```python
from build123d import *

# Parameters (mm, degrees)
SKETCH_1_W          = 124
SKETCH_1_H          = 65
EXTRUDE_1_DEPTH     = 18.5
SKETCH_2_R          = 1.5
CUT_EXTRUDE_1_DEPTH = 3
SKETCH_3_W          = 14
SKETCH_3_H          = 7
SKETCH_3_W_2        = 12
SKETCH_3_H_2        = 2
CUT_EXTRUDE_2_DEPTH = 3
SKETCH_4_R          = 0.5
CUT_EXTRUDE_3_DEPTH = 3
FILLET_1_R          = 2
FILLET_2_R          = 2
FILLET_3_R          = 2
FILLET_4_R          = 2


with BuildPart() as part:
    # Эскиз1 → Бобышка-Вытянуть1 (new body)
    with BuildSketch(Plane(origin=(0, 0, 0), x_dir=(1, 0, 0), z_dir=(0, 1, 0))):
        with Locations((62, 32.5)):
            Rectangle(SKETCH_1_W, SKETCH_1_H)
    extrude(amount=EXTRUDE_1_DEPTH)

    # Эскиз2 → Вырез-Вытянуть1 (cut)
    with BuildSketch(Plane(origin=(124, 0, 0), x_dir=(0, 0, -1), z_dir=(1, 0, 0))):
        with BuildLine():
            Line((11, 14.25), (21, 14.25))
            ThreePointArc((21, 14.25), (26, 9.25), (21, 4.25))
            Line((21, 4.25), (11, 4.25))
            ThreePointArc((11, 4.25), (6, 9.25), (11, 14.25))
        make_face()
        with Locations((11, 9.25)):
            Circle(SKETCH_2_R, mode=Mode.SUBTRACT)
        with Locations((21, 9.25)):
            Circle(SKETCH_2_R, mode=Mode.SUBTRACT)
    extrude(amount=-CUT_EXTRUDE_1_DEPTH, mode=Mode.SUBTRACT)

    # Эскиз3 → Вырез-Вытянуть2 (cut)
    with BuildSketch(Plane.ZY):
        with Locations((-52, 9.25)):
            Rectangle(SKETCH_3_W, SKETCH_3_H)
        with Locations((-52, 7.75)):
            Rectangle(SKETCH_3_W_2, SKETCH_3_H_2, mode=Mode.SUBTRACT)
    extrude(amount=-CUT_EXTRUDE_2_DEPTH, mode=Mode.SUBTRACT)

    # Эскиз4 → Вырез-Вытянуть3 (cut)
    with BuildSketch(Plane.ZY):
        Polygon((-19, 9.25), (-16, 12.25), (-10, 12.25), (-7, 9.25), (-10, 6.25), (-16, 6.25), align=None)
        with Locations((-16, 9.25)):
            Circle(SKETCH_4_R, mode=Mode.SUBTRACT)
        with Locations((-14, 9.25)):
            Circle(SKETCH_4_R, mode=Mode.SUBTRACT)
        with Locations((-12, 9.25)):
            Circle(SKETCH_4_R, mode=Mode.SUBTRACT)
        with Locations((-10, 9.25)):
            Circle(SKETCH_4_R, mode=Mode.SUBTRACT)
    extrude(amount=-CUT_EXTRUDE_3_DEPTH, mode=Mode.SUBTRACT)

    # Скругление1
    fillet_1_edges = [part.edges().sort_by_distance(p)[0] for p in [
        (124, 18.5, -32.5),
        (62, 18.5, -65),
        (0, 18.5, -32.5),
        (62, 18.5, 0),
    ]]
    fillet(fillet_1_edges, radius=FILLET_1_R)

    # Скругление2
    fillet_2_edges = [part.edges().sort_by_distance(p)[0] for p in [
        (62, 0, -65),
        (124, 0, -32.5),
        (62, 0, 0),
        (0, 0, -32.5),
    ]]
    fillet(fillet_2_edges, radius=FILLET_2_R)

    # Скругление3
    # the kernel refuses this fillet: 2 mm, written as the material it takes off along each edge
    with BuildSketch(Plane(origin=(2, 16.5, -2), x_dir=(-1, 0, 0), z_dir=(0, 0, 1))) as fillet_3_piece_1_section:
        Polygon((0, 0), (FILLET_3_R, 0), (FILLET_3_R, -FILLET_3_R), (0, -FILLET_3_R), align=None)
    fillet_3_piece_1 = extrude(amount=FILLET_3_R, mode=Mode.PRIVATE)
    fillet_3_piece_1 = fillet_3_piece_1 - Plane(origin=(2, 16.5, -2), x_dir=(0.7071067811865475, -0.7071067811865475, 0), z_dir=(0, 0, 1)) * Sphere(FILLET_3_R, mode=Mode.PRIVATE)
    add(fillet_3_piece_1, mode=Mode.SUBTRACT)
    with BuildSketch(Plane(origin=(122, 16.5, -2), x_dir=(1, 0, 0), z_dir=(0, 0, 1))) as fillet_3_piece_2_section:
        Polygon((0, 0), (FILLET_3_R, 0), (FILLET_3_R, FILLET_3_R), (0, FILLET_3_R), align=None)
    fillet_3_piece_2 = extrude(amount=FILLET_3_R, mode=Mode.PRIVATE)
    fillet_3_piece_2 = fillet_3_piece_2 - Plane(origin=(122, 16.5, -2), x_dir=(-0.7071067811865475, -0.7071067811865475, 0), z_dir=(0, 0, 1)) * Sphere(FILLET_3_R, mode=Mode.PRIVATE)
    add(fillet_3_piece_2, mode=Mode.SUBTRACT)
    with BuildSketch(Plane(origin=(2, 2, -2), x_dir=(-1, 0, 0), z_dir=(0, 0, 1))) as fillet_3_piece_3_section:
        Polygon((0, 0), (FILLET_3_R, 0), (FILLET_3_R, FILLET_3_R), (0, FILLET_3_R), align=None)
    fillet_3_piece_3 = extrude(amount=FILLET_3_R, mode=Mode.PRIVATE)
    fillet_3_piece_3 = fillet_3_piece_3 - Plane(origin=(2, 2, -2), x_dir=(0.7071067811865475, 0.7071067811865475, 0), z_dir=(0, 0, 1)) * Sphere(FILLET_3_R, mode=Mode.PRIVATE)
    add(fillet_3_piece_3, mode=Mode.SUBTRACT)
    with BuildSketch(Plane(origin=(122, 2, -2), x_dir=(1, 0, 0), z_dir=(0, 0, 1))) as fillet_3_piece_4_section:
        Polygon((0, 0), (FILLET_3_R, 0), (FILLET_3_R, -FILLET_3_R), (0, -FILLET_3_R), align=None)
    fillet_3_piece_4 = extrude(amount=FILLET_3_R, mode=Mode.PRIVATE)
    fillet_3_piece_4 = fillet_3_piece_4 - Plane(origin=(122, 2, -2), x_dir=(-0.7071067811865475, 0.7071067811865475, 0), z_dir=(0, 0, 1)) * Sphere(FILLET_3_R, mode=Mode.PRIVATE)
    add(fillet_3_piece_4, mode=Mode.SUBTRACT)
    with BuildSketch(Plane(origin=(124, 2, 0), x_dir=(-1, 0, 0), z_dir=(0, 1, 0))) as fillet_3_piece_5:
        with BuildLine():
            CenterArc((FILLET_3_R, -FILLET_3_R), FILLET_3_R, 90, 90)
            Line((0, -FILLET_3_R), (0, 0))
            Line((0, 0), (FILLET_3_R, 0))
        make_face()
    extrude(amount=14.5, mode=Mode.SUBTRACT)
    with BuildSketch(Plane(origin=(0, 2, 0), x_dir=(1, 0, 0), z_dir=(0, 1, 0))) as fillet_3_piece_6:
        with BuildLine():
            CenterArc((FILLET_3_R, FILLET_3_R), FILLET_3_R, 180, 90)
            Line((0, FILLET_3_R), (0, 0))
            Line((0, 0), (FILLET_3_R, 0))
        make_face()
    extrude(amount=14.5, mode=Mode.SUBTRACT)

    # Скругление4
    # the kernel refuses this fillet: 2 mm, written as the material it takes off along each edge
    with BuildSketch(Plane(origin=(2, 16.5, -63), x_dir=(0, 0, -1), z_dir=(-1, 0, 0))) as fillet_4_piece_1_section:
        Polygon((0, 0), (FILLET_4_R, 0), (FILLET_4_R, -FILLET_4_R), (0, -FILLET_4_R), align=None)
    fillet_4_piece_1 = extrude(amount=FILLET_4_R, mode=Mode.PRIVATE)
    fillet_4_piece_1 = fillet_4_piece_1 - Plane(origin=(2, 16.5, -63), x_dir=(0, -0.7071067811865475, 0.7071067811865475), z_dir=(-1, 0, 0)) * Sphere(FILLET_4_R, mode=Mode.PRIVATE)
    add(fillet_4_piece_1, mode=Mode.SUBTRACT)
    with BuildSketch(Plane(origin=(122, 16.5, -63), x_dir=(0, 0, -1), z_dir=(1, 0, 0))) as fillet_4_piece_2_section:
        Polygon((0, 0), (FILLET_4_R, 0), (FILLET_4_R, FILLET_4_R), (0, FILLET_4_R), align=None)
    fillet_4_piece_2 = extrude(amount=FILLET_4_R, mode=Mode.PRIVATE)
    fillet_4_piece_2 = fillet_4_piece_2 - Plane(origin=(122, 16.5, -63), x_dir=(0, -0.7071067811865475, 0.7071067811865475), z_dir=(1, 0, 0)) * Sphere(FILLET_4_R, mode=Mode.PRIVATE)
    add(fillet_4_piece_2, mode=Mode.SUBTRACT)
    with BuildSketch(Plane(origin=(2, 2, -63), x_dir=(0, 0, -1), z_dir=(-1, 0, 0))) as fillet_4_piece_3_section:
        Polygon((0, 0), (FILLET_4_R, 0), (FILLET_4_R, FILLET_4_R), (0, FILLET_4_R), align=None)
    fillet_4_piece_3 = extrude(amount=FILLET_4_R, mode=Mode.PRIVATE)
    fillet_4_piece_3 = fillet_4_piece_3 - Plane(origin=(2, 2, -63), x_dir=(0, 0.7071067811865475, 0.7071067811865475), z_dir=(-1, 0, 0)) * Sphere(FILLET_4_R, mode=Mode.PRIVATE)
    add(fillet_4_piece_3, mode=Mode.SUBTRACT)
    with BuildSketch(Plane(origin=(122, 2, -63), x_dir=(0, 0, -1), z_dir=(1, 0, 0))) as fillet_4_piece_4_section:
        Polygon((0, 0), (FILLET_4_R, 0), (FILLET_4_R, -FILLET_4_R), (0, -FILLET_4_R), align=None)
    fillet_4_piece_4 = extrude(amount=FILLET_4_R, mode=Mode.PRIVATE)
    fillet_4_piece_4 = fillet_4_piece_4 - Plane(origin=(122, 2, -63), x_dir=(0, 0.7071067811865475, 0.7071067811865475), z_dir=(1, 0, 0)) * Sphere(FILLET_4_R, mode=Mode.PRIVATE)
    add(fillet_4_piece_4, mode=Mode.SUBTRACT)
    with BuildSketch(Plane(origin=(124, 2, -65), x_dir=(0, 0, 1), z_dir=(0, 1, 0))) as fillet_4_piece_5:
        with BuildLine():
            CenterArc((FILLET_4_R, -FILLET_4_R), FILLET_4_R, 90, 90)
            Line((0, -FILLET_4_R), (0, 0))
            Line((0, 0), (FILLET_4_R, 0))
        make_face()
    extrude(amount=14.5, mode=Mode.SUBTRACT)
    with BuildSketch(Plane(origin=(0, 2, -65), x_dir=(0, 0, 1), z_dir=(0, 1, 0))) as fillet_4_piece_6:
        with BuildLine():
            CenterArc((FILLET_4_R, FILLET_4_R), FILLET_4_R, 180, 90)
            Line((0, FILLET_4_R), (0, 0))
            Line((0, 0), (FILLET_4_R, 0))
        make_face()
    extrude(amount=14.5, mode=Mode.SUBTRACT)


solid = part.part
```
For this review, take the finished solid that the model builds, in its own axes (mm). A direction names the side the tool comes from. Round coordinates to 2 decimals unless told otherwise and drop trailing zeros. Use one line per item in the form item = value.
Q1. To check wall thickness, follow probe 1 along X at (y, z) = (8.75, -13); probe 2 along X at (y, z) = (10.75, -47); probe 3 along Z at (x, y) = (51.5, 1.75). State the ranges of each line that lie inside material, in increasing order. Write a range as from..to.
Resolved:
probe_1 = 3..121
probe_2 = 3..124
probe_3 = -64.98..-0.02
Q2. Clearance check with flat-ended pins moving along their axes: pin 1 Ø0.6 at (x, y) = (1.5, 8) entering from -Z; pin 2 Ø1.5 at (x, z) = (1, -14) entering from +Y. State where each tip first meets the part, or that it passes through.
Resolved:
pin_1 = -64.99
pin_2 = 18.48
Q3. Machinability: for faces 4 (the flat face through (61, 0, -33)), 5 (the cylindrical face through (122.52, 9.14, -6)), 6 (the flat face through (1.48, 7.77, -8.48)), which of the approach directions +Z, -Z, +X, -X, +Y, -Y give a long, thin tool a straight path to every point of the face, cutting with its end or side? Answer none if there is none.
Resolved:
face_4 = +Z, -Z, +X, -X, -Y
face_5 = +X
face_6 = -X
Q4. The part is to be moulded in two halves that separate along Z. For faces 1 (the flat face through (1, 9, -45)), 2 (the flat face through (124, 9, -21)), 3 (the flat face through (61, 9, -65)), say which applies: released by +Z, released by -Z, zero draft, split by the parting line, or undercut.
Resolved:
face_1 = undercut
face_2 = zero draft
face_3 = released by -Z
